Source: CAD feature listing. Evaluate the final solid. Frame: model axes, mm. Face numbers are marked on the shaded views. A direction names the side the tool comes from. Round coordinates to 2 decimals unless told otherwise and drop trailing zeros. Loops run counter-clockwise (first coordinate to the right, second up) from the corner with the lowest first, then second, coordinate; pieces in that order, holes last. Notation, with made-up numbers: (1.25, 49) -> (29.25, 49) arc R24 ccw to (29.25, 75) -> close; hole circle Ø1 at (73, 41.5). An arc over 180 degrees is marked (long way). Write item = value, one per line.
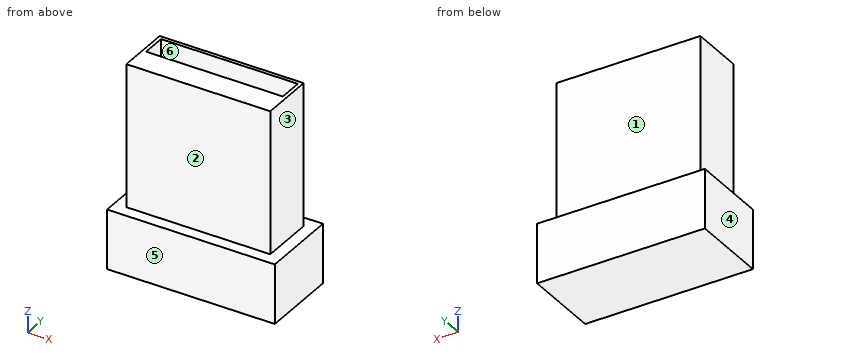
from build123d import *

# Parameters (mm, degrees)
F0_W     = 12.1
F0_H     = 4.5
F0_W_2   = 11.5
F0_H_2   = 3.9
F1_DEPTH = 12
F2_W     = 11.5
F2_H     = 1.88
F3_DEPTH = 12
F4_W     = 14.16
F4_H     = 6.56
F4_W_2   = 12.1
F4_H_2   = 4.5
F5_DEPTH = 5
F7_W     = 14.1
F7_H     = 6.5
F8_DEPTH = 5


with BuildPart() as f1:
    # F0 (on Top) → F1 (new body)
    with BuildSketch(Plane.XY):
        with Locations((6.05, 2.25)):
            Rectangle(F0_W, F0_H)
        with Locations((6.05, 2.25)):
            Rectangle(F0_W_2, F0_H_2, mode=Mode.SUBTRACT)
    extrude(amount=F1_DEPTH)

    # F2 (on Top) → F3 (join)
    with BuildSketch(Plane.XY):
        with Locations((6.05, 1.24)):
            Rectangle(F2_W, F2_H)
    extrude(amount=F3_DEPTH)

    # F7 (on face) → F8 (join)
    with BuildSketch(Plane(origin=(0, 0, 0), x_dir=(1, 0, 0), z_dir=(0, 0, -1))):
        with Locations((6.05, -2.25)):
            Rectangle(F7_W, F7_H)
    extrude(amount=F8_DEPTH)


with BuildPart() as f5:
    # F4 (on face) → F5 (new body)
    with BuildSketch(Plane(origin=(0, 0, 0), x_dir=(1, 0, 0), z_dir=(0, 0, -1))):
        with Locations((6.05, -2.25)):
            Rectangle(F4_W, F4_H)
        with Locations((6.05, -2.25)):
            Rectangle(F4_W_2, F4_H_2, mode=Mode.SUBTRACT)
    extrude(amount=F5_DEPTH)


solid = f1.part
1. Section query A-A (y = 0.25). Return the cut outline in (x, z).
Evaluation:
outline = (-1, -5) -> (13.1, -5) -> (13.1, 0) -> (12.1, 0) -> (12.1, 12) -> (0, 12) -> (0, 0) -> (-1, 0) -> close
2. Section query D-D (y = 2.5). Return the cut outline in (x, z), then the cut area to 3 significant figures.
Evaluation:
outline = (-1, -5) -> (13.1, -5) -> (13.1, 0) -> (12.1, 0) -> (12.1, 12) -> (11.8, 12) -> (11.8, 0) -> (0.3, 0) -> (0.3, 12) -> (0, 12) -> (0, 0) -> (-1, 0) -> close
area = 77.7 mm²
3. Section query B-B (z = 0.75). Return the cut outline in (x, y), then the cut area to 3 significant figures.
Evaluation:
outline = (0, 0) -> (12.1, 0) -> (12.1, 4.5) -> (0, 4.5) -> close; hole (0.3, 2.18) -> (11.8, 2.18) -> (11.8, 4.2) -> (0.3, 4.2) -> close
area = 31.2 mm²
4. Section query C-C (x = 3.5). Return the cut outline in (y, z), then the cut area to 3 significant figures.
Evaluation:
outline = (-1, -5) -> (5.5, -5) -> (5.5, 0) -> (4.5, 0) -> (4.5, 12) -> (4.2, 12) -> (4.2, 0) -> (2.18, 0) -> (2.18, 12) -> (0, 12) -> (0, 0) -> (-1, 0) -> close
area = 62.3 mm²
5. Mould query, pull axis Y, two halves, no side actions, for the marked faces 4, 5 and 6. Classes: released by +Y, released by -Y, zero draft, split by the parting line, or undercut.
Evaluation:
face_4 = zero draft
face_5 = released by -Y
face_6 = undercut
6. Line query: probe 1 along X at (y, z) = (3, 6.5); probe 2 along Y at (x, z) = (10.75, 2); probe 3 along Z at (x, y) = (6.5, 2.5). Output: solid intervals per line, ascending. Write a range as from..to.
Evaluation:
probe_1 = 0..0.3, 11.8..12.1
probe_2 = 0..2.18, 4.2..4.5
probe_3 = -5..0
7. Contact query for flat-ended pins moving along their axis: pin 1 Ø3.5 at (y, z) = (1, 5) entering from +X; pin 2 Ø1 at (x, y) = (5.5, 3) entering from +Z; pin 3 Ø3.5 at (y, z) = (2.5, 5) entering from -X. Output: stop coordinate, or through.
Evaluation:
pin_1 = 12.1
pin_2 = 0
pin_3 = 0
8. Set-up query: the marked faces 1, 2 and 3. Return all of +Z, -Z, +X, -X, +Y, -Y with unobstructed straight access to the full face (end or side cutting, diameter ignored); none if empty.
Evaluation:
face_1 = +Z, +X, -X, +Y
face_2 = +Z, +X, -X, -Y
face_3 = +Z, +X, +Y, -Y
